Autodesk Inventor part; units mm, degrees
ref_plane "YZ Plane" through (0, 0, 0) normal (1, 0, 0) x (0, 1, 0)
ref_plane "XZ Plane" through (0, 0, 0) normal (0, 1, 0) x (-1, 0, 0)
ref_plane "XY Plane" through (0, 0, 0) normal (0, 0, 1) x (1, 0, 0)
sketch "Sketch1" plane through (0, 0, 0) normal (0, 1, 0) x (-1, 0, 0)
  circle A0 centre (0, 0) radius 19.05
  dimension "d0" = 38.1
extrude "Extrusion1" add sketch "Sketch1" along normal blind 25.4
sketch "Sketch2" plane through (0, 25.4, 0) normal (0, 1, 0) x (1, 0, 0)
  circle A0 centre (0, 0) radius 3.175
  dimension "d3" = 6.35
extrude "Extrusion2" add sketch "Sketch2" along normal blind 12.7
extrude "Extrusion3" add sketch "Sketch2" against normal blind 38.1
sketch "Sketch3" plane through (0, 38.1, 0) normal (0, 1, 0) x (1, 0, 0)
  circle A0 centre (0, 0) radius 12.7
  dimension "d8" = 25.4
extrude "Extrusion4" add sketch "Sketch3" along normal blind 3.175
sketch "Sketch4" plane through (0, -12.7, 0) normal (0, -1, 0) x (1, 0, 0)
  circle A0 centre (0, 0) radius 12.7
  dimension "d11" = 25.4
extrude "Extrusion5" add sketch "Sketch4" along normal blind 3.175
properties part number "Gear Wheel"
The model under review builds one solid part; all positions refer to its coordinate system, in mm. A direction names the side the tool comes from. Round coordinates to 2 decimals unless told otherwise and drop trailing zeros. Write each loop counter-clockwise with the first axis right and the second up, starting at its lowest first coordinate (ties: lowest second). Pieces come first, ordered by that corner, then holes. Notation, with made-up numbers: M -23,80.5 L 22,80.5 A36 cw 22,118.5 Z; hole C 51,84.25 d7. An arc over 180 degrees is marked long. Use a Markdown table: item, result. Add a question column.
Q1. We need section A-A, the plane z = -9.5. State the section outline as (x, y) points (3 decimals).
Q2. Insertion check: pin 1 (6 mm diameter, centred on y = 29.5, z = 6.5, fed in from -X); pin 2 (5 mm diameter, centred on x = -12, z = -12, fed in from -Y); pin 3 (6 mm diameter, centred on x = 5.5, y = -1, fed in from -Z); pin 4 (12 mm diameter, centred on y = 5, z = -5.5, fed in from -X). Each pin has a flat end and moves straight along its axis. Give the tip position at first contact, or say it passes through.
Q3. We need section B-B, the plane x = 0. State the section outline as (y, z) points (3 decimals), plus the area to 3 significant figures.
Q4. To check wall thickness, follow line 1 (Y direction, x = 7.5, z = 7.5) (3 decimals); line 2 (Y direction, x = 2, z = 16); line 3 (Z direction, x = -11, y = 15.5). State the ranges of each line that lie inside material, in increasing order.
Q5. We need section D-D, the plane y = 24.5. State the section outline as (x, z) points, plus the area to 3 significant figures.
Q6. We need section C-C, the plane z = 0. State the section outline as (x, y) points (3 decimals).
Q7. The part is to be moulded in two halves that separate along Y. For faces 4 (the face through (0, -15.875, 0)), 5 (the face through (-4, 25.4, 0)), 6 (the face through (-2.75, 39.67, -12.4)), say which applies: pulls with the +Y half, pulls with the -Y half, needs draft (parallel to the pull), parting line crosses it, or undercut.
Q8. Machinability: for faces 1 (the face through (-0.69, 31.66, -3.1)), 2 (the face through (0, 41.275, 0)), 3 (the face through (-2.75, -14.27, 12.4)), which of the approach directions +Z, -Z, +X, -X, +Y, -Y give a long, thin tool a straight path to every point of the face, cutting with its end or side? Answer none if there is none.
Findings below:
| question | item | result |
|---|---|---|
| 1 | outline | M -16.512,0 L 16.512,0 L 16.512,25.4 L -16.512,25.4 Z; M -8.429,-15.875 L 8.429,-15.875 L 8.429,-12.7 L -8.429,-12.7 Z; M -8.429,38.1 L 8.429,38.1 L 8.429,41.275 L -8.429,41.275 Z |
| 2 | pin 1 | passes through |
| 2 | pin 2 | stops at y = 0 |
| 2 | pin 3 | stops at z = -18.86 |
| 2 | pin 4 | stops at x = -19.05 |
| 3 | outline | M -15.875,-12.7 L -12.7,-12.7 L -12.7,-3.175 L 0,-3.175 L 0,-19.05 L 25.4,-19.05 L 25.4,-3.175 L 38.1,-3.175 L 38.1,-12.7 L 41.275,-12.7 L 41.275,12.7 L 38.1,12.7 L 38.1,3.175 L 25.4,3.175 L 25.4,19.05 L 0,19.05 L 0,3.175 L -12.7,3.175 L -12.7,12.7 L -15.875,12.7 Z |
| 3 | area | 1,290 mm² |
| 4 | line 1 | y = -15.875 to -12.7, 0 to 25.4, 38.1 to 41.275 |
| 4 | line 2 | y = 0 to 25.4 |
| 4 | line 3 | z = -15.55 to 15.55 |
| 5 | outline | C 0,0 d38.1 |
| 5 | area | 1,140 mm² |
| 6 | outline | M -19.05,0 L -3.175,0 L -3.175,-12.7 L -12.7,-12.7 L -12.7,-15.875 L 12.7,-15.875 L 12.7,-12.7 L 3.175,-12.7 L 3.175,0 L 19.05,0 L 19.05,25.4 L 3.175,25.4 L 3.175,38.1 L 12.7,38.1 L 12.7,41.275 L -12.7,41.275 L -12.7,38.1 L -3.175,38.1 L -3.175,25.4 L -19.05,25.4 Z |
| 7 | face 4 | pulls with the -Y half |
| 7 | face 5 | undercut |
| 7 | face 6 | needs draft |
| 8 | face 1 | none |
| 8 | face 2 | +Z, -Z, +X, -X, +Y |
| 8 | face 3 | -Y |
